Geometry check sheet. Reference: the model listing, model coordinates, mm. Round coordinates to 2 decimals unless told otherwise and drop trailing zeros. Order: outer loops, then holes, each group sorted by start corner. A loop starts at its lowest first (then second) coordinate and runs counter-clockwise, first axis right, second up.
(1) Release check for a two-part mould opening along Z. For faces 1 (the face through (2.84, -0.74, -1.586)), 2 (the face through (67.69, -0.74, -7.16)), 3 (the face through (40, -1, -20.32)), 4 (the face through (40, -1, 0)) record: +Z half, -Z half, draft (parallel to the pull), parting line (faces both ways), or undercut.
(2) Sectioned sample at A-A (z = -2.54). Record the boundary of the cut face in (x, y).
(3) Material ranges on line 1 along X through (y, z) = (-0.3, -7.62); line 2 along Z through (x, y) = (78.74, -0.3); line 3 along X through (y, z) = (-0.8, -17.78), recorded low to high.
from build123d import *

# Parameters (mm, degrees)
SKETCH1_W           = 81.28
SKETCH1_H           = 20.32
SKETCH1_R           = 1
BOSS_EXTRUDE1_DEPTH = 1.5
SKETCH1_3_R         = 0.5
CUT_EXTRUDE1_DEPTH  = 0.762


with BuildPart() as part:
    # Sketch1 → Boss-Extrude1 (new body)
    with BuildSketch(Plane(origin=(0, 0, 0), x_dir=(1, 0, 0), z_dir=(0, 1, 0))):
        with Locations((40.64, 10.16)):
            Rectangle(SKETCH1_W, SKETCH1_H)
        with Locations(Location((2.54, 2.54, 0), (0, 0, 270))):  # turned: the seam where the file's is
            Circle(SKETCH1_R, mode=Mode.SUBTRACT)
        with Locations(Location((68.58, 7.62, 0), (0, 0, 270))):  # turned: the seam where the file's is
            Circle(SKETCH1_R, mode=Mode.SUBTRACT)
        with Locations(Location((2.54, 17.78, 0), (0, 0, 270))):  # turned: the seam where the file's is
            Circle(SKETCH1_R, mode=Mode.SUBTRACT)
    extrude(amount=-BOSS_EXTRUDE1_DEPTH)

    # Sketch1_3 → Cut-Extrude1 (cut)
    with BuildSketch(Plane(origin=(0, 0, 0), x_dir=(1, 0, 0), z_dir=(0, 1, 0))):
        with Locations(Location((2.54, 12.7, 0), (0, 0, 270))):  # turned: the seam where the file's is
            Circle(SKETCH1_3_R)
        with Locations(Location((2.54, 10.16, 0), (0, 0, 270))):  # turned: the seam where the file's is
            Circle(SKETCH1_3_R)
        with Locations(Location((78.74, 7.62, 0), (0, 0, 270))):  # turned: the seam where the file's is
            Circle(SKETCH1_3_R)
        with Locations(Location((78.74, 10.16, 0), (0, 0, 270))):  # turned: the seam where the file's is
            Circle(SKETCH1_3_R)
    extrude(amount=-CUT_EXTRUDE1_DEPTH, mode=Mode.SUBTRACT)


solid = part.part
Answer below:
1. face 1: undercut
1. face 2: undercut
1. face 3: -Z half
1. face 4: +Z half
2. outline: (0, -1.5) - (1.54, -1.5) - (1.54, 0) - (0, 0) - close; (3.54, -1.5) - (81.28, -1.5) - (81.28, 0) - (3.54, 0) - close
3. line 1: x = 0 to 67.58, 69.58 to 78.24, 79.24 to 81.28
3. line 2: z = -20.32 to -10.66, -9.66 to -8.12, -7.12 to 0
3. line 3: x = 0 to 1.54, 3.54 to 81.28
